Source: CAD feature listing. Evaluate the final solid. Frame: model axes, mm. A direction names the side the tool comes from. Coordinates: 2 decimals unless noted, no trailing zeros. Order: outer loops, then holes, each group sorted by start corner. A loop starts at its lowest first (then second) coordinate and runs counter-clockwise, first axis right, second up. Notation, with made-up numbers: (13.5, -35.75) -> (24.5, -35.75) arc R19 cw to (24.5, -22.75) -> close; hole circle Ø9 at (7, 74.25). An arc over 180 degrees is marked (long way). Put each result on its own line as item: value.
from build123d import *

# Parameters (mm, degrees)
F0_R     = 2.55
F0_R_2   = 12.5
F1_DEPTH = 6


with BuildPart() as f1:
    # F0 (on Top) → F1 (new body)
    with BuildSketch(Plane.XY):
        with BuildLine():
            ThreePointArc((19.5959179423, 19), (16.6682177234, 19.4381711253), (13.9970842445, 20.7142857143))
            ThreePointArc((13.9970842445, 20.7142857143), (-25, 0), (13.9970842445, -20.7142857143))
            ThreePointArc((13.9970842445, -20.7142857143), (16.6682177234, -19.4381711253), (19.5959179423, -19))
            Line((19.5959179423, -19), (75, -19))
            ThreePointArc((75, -19), (83.3493660836, -17.0671639707), (90, -11.6619037897))
            Line((90, -11.6619037897), (90, 11.6619037897))
            ThreePointArc((90, 11.6619037897), (83.3493660836, 17.0671639707), (75, 19))
            Line((75, 19), (19.5959179423, 19))
        make_face()
        with Locations((-14.4956890143, -14.4956890143)):
            Circle(F0_R, mode=Mode.SUBTRACT)
        with Locations((14.4956890143, -14.4956890143)):
            Circle(F0_R, mode=Mode.SUBTRACT)
        with BuildLine():
            ThreePointArc((61.1611652352, -10.4388347648), (59.5611652352, -8.8388347648), (61.1611652352, -7.2388347648))
            Line((61.1611652352, -7.2388347648), (66.1611652352, -7.2388347648))
            ThreePointArc((66.1611652352, -7.2388347648), (67.7611652352, -8.8388347648), (66.1611652352, -10.4388347648))
            Line((66.1611652352, -10.4388347648), (61.1611652352, -10.4388347648))
        make_face(mode=Mode.SUBTRACT)
        with BuildLine():
            ThreePointArc((78.8388347648, -10.4388347648), (77.2388347648, -8.8388347648), (78.8388347648, -7.2388347648))
            Line((78.8388347648, -7.2388347648), (83.8388347648, -7.2388347648))
            ThreePointArc((83.8388347648, -7.2388347648), (85.4388347648, -8.8388347648), (83.8388347648, -10.4388347648))
            Line((83.8388347648, -10.4388347648), (78.8388347648, -10.4388347648))
        make_face(mode=Mode.SUBTRACT)
        Circle(F0_R_2, mode=Mode.SUBTRACT)
        with Locations((-14.4956890143, 14.4956890143)):
            Circle(F0_R, mode=Mode.SUBTRACT)
        with Locations((14.4956890143, 14.4956890143)):
            Circle(F0_R, mode=Mode.SUBTRACT)
        with BuildLine():
            ThreePointArc((61.1611652352, 7.2388347648), (59.5611652352, 8.8388347648), (61.1611652352, 10.4388347648))
            Line((61.1611652352, 10.4388347648), (66.1611652352, 10.4388347648))
            ThreePointArc((66.1611652352, 10.4388347648), (67.7611652352, 8.8388347648), (66.1611652352, 7.2388347648))
            Line((66.1611652352, 7.2388347648), (61.1611652352, 7.2388347648))
        make_face(mode=Mode.SUBTRACT)
        with BuildLine():
            ThreePointArc((70, -6.75), (63.25, 0), (70, 6.75))
            Line((70, 6.75), (75, 6.75))
            ThreePointArc((75, 6.75), (81.75, 0), (75, -6.75))
            Line((75, -6.75), (70, -6.75))
        make_face(mode=Mode.SUBTRACT)
        with BuildLine():
            ThreePointArc((78.8388347648, 7.2388347648), (77.2388347648, 8.8388347648), (78.8388347648, 10.4388347648))
            Line((78.8388347648, 10.4388347648), (83.8388347648, 10.4388347648))
            ThreePointArc((83.8388347648, 10.4388347648), (85.4388347648, 8.8388347648), (83.8388347648, 7.2388347648))
            Line((83.8388347648, 7.2388347648), (78.8388347648, 7.2388347648))
        make_face(mode=Mode.SUBTRACT)
        with BuildLine():
            ThreePointArc((90, -11.6619037897), (94, 0), (90, 11.6619037897))
            Line((90, 11.6619037897), (90, -11.6619037897))
        make_face()
    extrude(amount=F1_DEPTH)


solid = f1.part
1. Pull-direction query (X, two-part tool) for faces 3 (the flat face through (64, 10.439, 3)), 4 (the cylindrical face through (16.708, 19.426, 2.958)), 5 (the flat face through (47, -19, 3)); classes: pulls with the +X half, pulls with the -X half, needs draft (parallel to the pull), parting line crosses it, or undercut.
Numbers:
face 3: undercut
face 4: pulls with the +X half
face 5: needs draft
2. Cut plane D-D on x = 37.5. Output: boundary loops of the cut face in (y, z).
Numbers:
outline: (-19, 0) -> (19, 0) -> (19, 6) -> (-19, 6) -> close
3. Cut plane C-C on z = 3.15. Count the separate pieces of the cut face and the enclosed holes in it, plus the area to 3 significant figures.
Numbers:
separate pieces: 1
enclosed holes: 10
area: 3,660 mm2
4. Cut plane A-A on y = 0. Output: boundary loops of the cut face in (x, z).
Numbers:
outline: (-25, 0) -> (-12.5, 0) -> (-12.5, 6) -> (-25, 6) -> close; (12.5, 0) -> (63.25, 0) -> (63.25, 6) -> (12.5, 6) -> close; (81.75, 0) -> (94, 0) -> (94, 6) -> (81.75, 6) -> close
5. Ray query, line 1 along Y through (x, z) = (63, 1.2); line 2 along X through (y, z) = (15, 5.05); line 3 along Y through (x, z) = (64, 3.65). Return the intervals inside material, ascending.
Numbers:
line 1: y = -19 to -10.44, -7.24 to 7.24, 10.44 to 19
line 2: x = -20 to -17, -12 to 12, 17 to 86.66
line 3: y = -19 to -10.44, -7.24 to -3.09, 3.09 to 7.24, 10.44 to 19
6. Cut plane B-B on x = 0. Output: boundary loops of the cut face in (y, z), plus the area to 3 significant figures.
Numbers:
outline: (-25, 0) -> (-12.5, 0) -> (-12.5, 6) -> (-25, 6) -> close; (12.5, 0) -> (25, 0) -> (25, 6) -> (12.5, 6) -> close
area: 150 mm2
7. First-contact query: pin 1 (1.5 mm diameter, centred on x = 44.5, z = 3, fed in from +Y); pin 2 (2.5 mm diameter, centred on x = 82, z = 1.5, fed in from +Y); pin 3 (3 mm diameter, centred on x = -14.5, y = -14.5, fed in from +Z); pin 4 (2.5 mm diameter, centred on x = 64, z = 2.5, fed in from -Y). Flat tips, straight axial feed; report the tip coordinate or a pass-through.
Numbers:
pin 1: stops at y = 19
pin 2: stops at y = 18.11
pin 3: passes through
pin 4: stops at y = -19
8. Set-up query: faces 1 (the flat face through (34, 0, 6)), 2 (the flat face through (81, 10.439, 3)). Return all of +Z, -Z, +X, -X, +Y, -Y with unobstructed straight access to the full face (end or side cutting, diameter ignored); none if empty.
Numbers:
face 1: +Z, +X, -X, +Y, -Y
face 2: +Z, -Z
